```python
from build123d import *

# Parameters (mm, degrees)
SKETCH1_W           = 90
SKETCH1_H           = 67
BOSS_EXTRUDE1_DEPTH = 40
SHELL1_T            = -2
SKETCH2_W           = 50
SKETCH2_H           = 13
CUT_EXTRUDE4_DEPTH  = 40
SKETCH4_W           = 54
SKETCH4_H           = 13
BOSS_EXTRUDE2_DEPTH = 75
SHELL2_START        = 11.213016769
SHELL2_OUTLINE_W    = 9
SHELL2_OUTLINE_H    = 73
SHELL2_DEPTH        = 50


# Read off the part's stored shape, not the designer's step: Shell2
with BuildPart() as part:
    # Sketch1 → Boss-Extrude1 (new, symmetric)
    with BuildSketch(Plane.XY.offset(58.585622103)):
        with Locations((36.213016769, 11.266964079)):
            Rectangle(SKETCH1_W, SKETCH1_H)
    extrude(amount=BOSS_EXTRUDE1_DEPTH, both=True)

    # Shell1
    shell1_openings = [part.faces().sort_by_distance(p)[0] for p in [
        (36.213016769, 44.766964079, 58.585622103),
    ]]
    offset(amount=SHELL1_T, openings=shell1_openings, kind=Kind.INTERSECTION)

    # Sketch2 → Cut-Extrude4 (cut)
    with BuildSketch(Plane.XY.offset(98.585622103)):
        with Locations((36.213016769, -12.733035921)):
            Rectangle(SKETCH2_W, SKETCH2_H)
    extrude(amount=-CUT_EXTRUDE4_DEPTH, mode=Mode.SUBTRACT)

    # Sketch4 → Boss-Extrude2 (add)
    with BuildSketch(Plane.XY.offset(98.585622103)):
        with Locations((36.213016769, -12.733035921)):
            Rectangle(SKETCH4_W, SKETCH4_H)
    extrude(amount=-BOSS_EXTRUDE2_DEPTH)

    # Shell2 outline → Shell2 (cut)
    with BuildSketch(Plane.YZ.offset(SHELL2_START)):
        with Locations((-12.733035921, 62.085622103)):
            Rectangle(SHELL2_OUTLINE_W, SHELL2_OUTLINE_H)
    extrude(amount=SHELL2_DEPTH, mode=Mode.SUBTRACT)


solid = part.part
```
Design review of the part built by this model. Coordinates are the model's own, in mm. A direction names the side the tool comes from. Give positions to 0.01 mm unless a question says otherwise; leave off trailing zeros. Order: outer loops, then holes, each group sorted by start corner. A loop starts at its lowest first (then second) coordinate and runs counter-clockwise, first axis right, second up. Notation, with made-up numbers: (86.25, -10) - (94.25, -10) arc R32 cw to (94.25, 17) - close; hole circle Ø7 at (-38, -0.5). An arc over 180 degrees is marked (long way). Use a Markdown table: item, result. Add a question column.
(1) Add section D-D on y = -11.5. Give the boundary of the cut face in (x, z), then the cut area to 3 significant figures.
(2) Clearance check with a flat-ended pin moving along its axis: P1, Ø10, axis at x = 42.5, z = 78.5, coming from the +Y side. State where the tip first meets the part, or that it passes through.
(3) Machinability: for faces 1 (the face through (63.213, -13, 61)), 2 (the face through (36, -19.233, 61)), 3 (the face through (36, -13, 25.586)), which of the approach directions +Z, -Z, +X, -X, +Y, -Y give a long, thin tool a straight path to every point of the face, cutting with its end or side? Answer none if there is none.
(4) Add section B-B on y = 35. Give the boundary of the cut face in (x, z).
(5) Wall thickness on probe 1 along Y at (x, z) = (28, 55.5); probe 2 along X at (y, z) = (-10, 35.5); probe 3 along Z at (x, y) = (55, 0.5): over which ranges is each line inside the solid? List them lowest first. Write a range as [from, to].
(6) Add section C-C on x = 24.5. Give the boundary of the cut face in (y, z), then the cut area to 3 significant figures.
(7) Add section A-A on z = 70.5. Give the boundary of the cut face in (x, y).
(8) Mouldability with a two-part tool opening along Y and no side actions: class faces 4 (the face through (36, -22.233, 59)), 5 (the face through (81.213, 11, 59)), 6 (the face through (36, -8.233, 62)) as +Y half, -Y half, draft (parallel to the pull), parting line (faces both ways), or undercut.
Report:
| question | item | result |
|---|---|---|
| 1 | outline | (-8.79, 18.59) - (81.21, 18.59) - (81.21, 98.59) - (61.21, 98.59) - (61.21, 25.59) - (11.21, 25.59) - (11.21, 98.59) - (-8.79, 98.59) - close; hole (-6.79, 20.59) - (79.21, 20.59) - (79.21, 96.59) - (63.21, 96.59) - (63.21, 23.59) - (9.21, 23.59) - (9.21, 96.59) - (-6.79, 96.59) - close |
| 1 | area | 956 mm² |
| 2 | P1 | stops at y = -6.23 |
| 3 | face 1 | +Y |
| 3 | face 2 | none |
| 3 | face 3 | +Z |
| 4 | outline | (-8.79, 18.59) - (81.21, 18.59) - (81.21, 98.59) - (-8.79, 98.59) - close; hole (-6.79, 20.59) - (79.21, 20.59) - (79.21, 96.59) - (-6.79, 96.59) - close |
| 5 | probe 1 | y = [-22.23, -20.23], [-19.23, -17.23], [-8.23, -6.23] |
| 5 | probe 2 | x = [-8.79, -6.79], [9.21, 11.21], [61.21, 63.21], [79.21, 81.21] |
| 5 | probe 3 | z = [18.59, 20.59], [96.59, 98.59] |
| 6 | outline | (-22.23, 18.59) - (44.77, 18.59) - (44.77, 20.59) - (-20.23, 20.59) - (-20.23, 96.59) - (-19.23, 96.59) - (-19.23, 23.59) - (-6.23, 23.59) - (-6.23, 96.59) - (44.77, 96.59) - (44.77, 98.59) - (-8.23, 98.59) - (-8.23, 25.59) - (-17.23, 25.59) - (-17.23, 98.59) - (-22.23, 98.59) - close |
| 6 | area | 712 mm² |
| 7 | outline | (-8.79, -22.23) - (81.21, -22.23) - (81.21, 44.77) - (79.21, 44.77) - (79.21, -20.23) - (-6.79, -20.23) - (-6.79, 44.77) - (-8.79, 44.77) - close; (9.21, -19.23) - (63.21, -19.23) - (63.21, -6.23) - (9.21, -6.23) - close; hole (11.21, -17.23) - (61.21, -17.23) - (61.21, -8.23) - (11.21, -8.23) - close |
| 8 | face 4 | -Y half |
| 8 | face 5 | draft |
| 8 | face 6 | undercut |
